Could you check a few things on this model? Use its own coordinates, in mm. Face numbers are marked on the shaded views. A direction names the side the tool comes from. Give positions to 0.01 mm unless a question says otherwise; leave off trailing zeros. One line per item, written item: value.
```python
from build123d import *

# Parameters (mm, degrees)
CUT_EXTRUDE2_OUTLINE_R = 47.625
CUT_EXTRUDE2_DEPTH     = 7.234682
F_10_CLEARANCE_HOLE1_D = 5.1054
CIRPATTERN1_COUNT      = 8
CLEARANCING_START      = -7.234682
SKETCH25_R             = 66.675
CLEARANCING_DEPTH      = 7.234682


# Read off the part's stored shape, not the designer's step: Cut-Extrude2
with BuildPart() as part:
    # Sketch24 → Revolve1 (revolve)
    with BuildSketch(Plane(origin=(0, 0, 0), x_dir=(1, 0, 0), z_dir=(0, 1, 0))):
        Polygon((-17.018, -22.86), (-17.018, -8.923782), (-34.42208, -8.923782), (-34.42208, 0), (-47.625, 0), (-47.625, -7.234682), (-46.0375, -7.234682), (-46.0375, -10.371582), (-50.8, -10.371582), (-50.8, -7.234682), (-66.675, -7.234682), (-66.675, -22.86), align=None)
    revolve(axis=Axis((0, 0, -9.275318), (0, 0, 1)))

    # Cut-Extrude2 outline → Cut-Extrude2 (cut)
    with BuildSketch(Plane.XY):
        Circle(CUT_EXTRUDE2_OUTLINE_R)
        with BuildLine():
            add(Edge.make_bspline(
                [(35.948703812, 0), (35.9515816, 0.07538119), (35.957337916, 0.226162951), (35.964207937, 0.452426553), (35.969771157, 0.678783022), (35.978029534, 1.131847853), (35.980843708, 2.190601907), (35.920311441, 3.779931016), (35.747323363, 5.668216834), (35.489928088, 7.474298946), (35.141459932, 9.268877369), (34.702390603, 11.047358984), (34.17343386, 12.80516853), (33.555538624, 14.537761538), (32.849887572, 16.240636382), (32.057893687, 17.909346365), (31.181197352, 19.53951152), (30.221662701, 21.126830276), (29.181373626, 22.667090912), (28.062629225, 24.156182809), (26.867938753, 25.590107465), (25.60001603, 26.964989265), (24.261773335, 28.277085961), (22.856314773, 29.522798851), (21.386929147, 30.698682629), (19.85708232, 31.801454876), (18.270409111, 32.828005175), (16.630704717, 33.775403815), (14.941915703, 34.640910073), (13.208130556, 35.421980041), (11.43356985, 36.116273987), (9.622576022, 36.721663214), (7.779602801, 37.236236415), (5.909204301, 37.658305492), (4.016023818, 37.986410831), (2.104782347, 38.219326014), (0.180266852, 38.356061949), (-1.75268168, 38.395870413), (-3.689180377, 38.338246992), (-5.624316777, 38.182933409), (-7.553161251, 37.929919231), (-9.470779522, 37.579442948), (-11.37224525, 37.131992419), (-13.252652651, 36.588304682), (-15.107129112, 35.949365124), (-16.930847778, 35.216406011), (-18.719040078, 34.390904381), (-20.467008144, 33.474579298), (-22.170137115, 32.469388481), (-23.823907266, 31.377524301), (-25.42390596, 30.201409162), (-26.965839357, 28.943690275), (-28.445543888, 27.607233836), (-29.858997424, 26.195118613), (-31.202330147, 24.710628968), (-32.471835063, 23.157247319), (-33.663978152, 21.538646066), (-34.775408104, 19.858679), (-35.802965645, 18.121372202), (-36.743692396, 16.330914471), (-37.594839261, 14.491647299), (-38.353874308, 12.608054401), (-39.018490139, 10.68475085), (-39.586610697, 8.726471825), (-40.056397525, 6.738061006), (-40.426255434, 4.724458642), (-40.694837576, 2.690689328), (-40.861049894, 0.641849508), (-40.924054953, -1.416905249), (-40.883275123, -3.480373184), (-40.738395114, -5.543319447), (-40.489363842, -7.600489337), (-40.13639564, -9.646621653), (-39.679970776, -11.676462103), (-39.120835312, -13.684776759), (-38.460000265, -15.666365517), (-37.698740094, -17.61607551), (-36.838590511, -19.528814477), (-35.881345602, -21.399564006), (-34.829054288, -23.223392663), (-33.684016107, -24.995468936), (-32.44877635, -26.711073982), (-31.126120537, -28.365614138), (-29.719068263, -29.954633155), (-28.230866416, -31.473824138), (-26.664981791, -32.919041144), (-25.025093105, -34.286310417), (-23.315082441, -35.571841228), (-21.53902614, -36.772036288), (-19.701185153, -37.883501708), (-17.805994889, -38.903056478), (-15.85805457, -39.827741435), (-13.862116128, -40.654827709), (-11.823072667, -41.381824596), (-9.745946518, -42.006486871), (-7.635876912, -42.526821485), (-5.498107312, -42.941093656), (-3.337972426, -43.247832311), (-1.160884928, -43.445834888), (1.027678058, -43.534171454), (3.222188708, -43.512188152), (5.417082419, -43.379509955), (7.606771886, -43.136042707), (9.785661288, -42.781974466), (11.948160555, -42.317776118), (14.08869967, -41.74420128), (16.201742982, -41.062285471), (18.281803484, -40.273344558), (20.323457017, -39.378972487), (22.321356376, -38.381038284), (24.27024527, -37.281682345), (26.164972102, -36.083312015), (28.000503535, -34.788596469), (29.77193781, -33.400460899), (31.474517775, -31.92208003), (33.103643596, -30.356870964), (34.654885111, -28.708485383), (36.123993806, -26.980801118), (37.506914359, -25.17791311), (38.799795742, -23.304123775), (39.999001844, -21.363932809), (41.101121576, -19.362026441), (41.938186302, -17.641904891), (42.402189205, -16.588613759), (42.554027377, -16.231646763)],
                knots=[0, 0, 0, 0, 0.000879209, 0.001758645, 0.002638305, 0.003518191, 0.007039982, 0.014977213, 0.022047939, 0.029133237, 0.036233164, 0.043347773, 0.050477114, 0.057621232, 0.06478017, 0.071953969, 0.079142669, 0.086346306, 0.093564916, 0.100798534, 0.108047194, 0.115310927, 0.122589766, 0.12988374, 0.13719288, 0.144517215, 0.151856774, 0.159211583, 0.16658167, 0.173967063, 0.181367786, 0.188783866, 0.196215328, 0.203662198, 0.211124498, 0.218602253, 0.226095488, 0.233604225, 0.241128486, 0.248668296, 0.256223676, 0.263794648, 0.271381234, 0.278983456, 0.286601335, 0.294234891, 0.301884146, 0.309549121, 0.317229835, 0.324926308, 0.332638561, 0.340366614, 0.348110485, 0.355870195, 0.363645762, 0.371437205, 0.379244543, 0.387067795, 0.39490698, 0.402762115, 0.410633219, 0.41852031, 0.426423405, 0.434342523, 0.442277682, 0.450228898, 0.458196189, 0.466179572, 0.474179065, 0.482194684, 0.490226447, 0.498274369, 0.506338468, 0.514418761, 0.522515263, 0.530627991, 0.538756962, 0.546902191, 0.555063694, 0.563241488, 0.571435588, 0.57964601, 0.58787277, 0.596115883, 0.604375364, 0.61265123, 0.620943495, 0.629252175, 0.637577285, 0.64591884, 0.654276855, 0.662651345, 0.671042324, 0.679449808, 0.687873812, 0.696314349, 0.704771435, 0.713245083, 0.721735309, 0.730242127, 0.738765551, 0.747305595, 0.755862273, 0.7644356, 0.77302559, 0.781632256, 0.790255613, 0.798895674, 0.807552454, 0.816225965, 0.824916222, 0.833623239, 0.842347028, 0.851087604, 0.859844979, 0.868619169, 0.877410184, 0.88621804, 0.895042749, 0.903884325, 0.912742781, 0.921618129, 0.930510383, 0.935031581, 0.935031581, 0.935031581, 0.935031581], degree=3))
            ThreePointArc((35.948703812, 0), (36.836858206, -3.871377871), (39.552581276, -6.769865934))
            ThreePointArc((39.552581276, -6.769865934), (42.805320101, -10.94498561), (42.554027377, -16.231646763))
        make_face(mode=Mode.SUBTRACT)
    extrude(amount=CUT_EXTRUDE2_DEPTH, mode=Mode.SUBTRACT)

    # #10 Clearance Hole1 (through all)
    with Locations(Plane(origin=(55.733032799, -23.085378057, 7.234682), x_dir=(-1, 0, 0), z_dir=(0, 0, -1))):
        with Locations((0, 0)):
            f_10_clearance_hole1 = Hole(F_10_CLEARANCE_HOLE1_D / 2)

    # CirPattern1: #10 Clearance Hole1 ×8 about axis
    cirpattern1_axis = Axis((0, 0, 0), (0, 0, 1))
    for i in range(1, CIRPATTERN1_COUNT):
        add(f_10_clearance_hole1.rotate(cirpattern1_axis, i * 360 / CIRPATTERN1_COUNT), mode=Mode.SUBTRACT)

    # Sketch25 → Clearancing (cut)
    with BuildSketch(Plane(origin=(0, 0, 0), x_dir=(-1, 0, 0), z_dir=(0, 0, -1)).offset(CLEARANCING_START)):
        Circle(SKETCH25_R)
        with BuildLine():
            ThreePointArc((-39.485738347, -6.87785215), (-42.684264858, -10.983386498), (-42.437160346, -16.181936632))
            add(Edge.make_bspline(
                [(-42.437160346, -16.181936632), (-41.450328446, -18.501948894), (-40.287188075, -20.70386066), (-37.62426385, -24.882183045), (-36.1244575, -26.858578596), (-33.612918368, -29.647784963), (-32.727511557, -30.551787217), (-30.899288351, -32.26713978), (-29.954285679, -33.081629815), (-27.028415852, -35.398073541), (-24.957331886, -36.773902575), (-22.214143518, -38.277928099), (-21.657736444, -38.567871448), (-20.529077868, -39.125607363), (-19.957869924, -39.392805227), (-18.236811973, -40.153613466), (-17.074606136, -40.608998857), (-13.544408375, -41.82291337), (-11.1331575, -42.430323242), (-8.045152005, -42.931279628), (-7.423828634, -43.018467653), (-6.17358737, -43.166313281), (-5.545687994, -43.226778512), (-3.668882092, -43.366672694), (-2.421130233, -43.405411027), (1.311985825, -43.361475459), (3.787286298, -43.119848136), (7.47956464, -42.43089353), (8.712476258, -42.144649273), (11.128372813, -41.470614218), (12.31452175, -41.08278751), (15.808874803, -39.769919796), (18.053477953, -38.696639775), (21.289209419, -36.780985477), (22.349089848, -36.088250708), (24.383348169, -34.625595136), (25.362502881, -33.853290457), (28.188051648, -31.415612474), (29.923427118, -29.630442917), (31.900539288, -27.191684875), (32.287236817, -26.69215724), (33.03483793, -25.679954076), (33.395921295, -25.167211132), (34.441621812, -23.609372602), (35.088773016, -22.544710991), (36.882357275, -19.273503621), (37.882174946, -16.990390194), (38.875744828, -14.00270068), (39.061155114, -13.399331831), (39.402369545, -12.191519857), (39.558676578, -11.585611614), (39.985275792, -9.761961138), (40.441402975, -7.314651304), (40.674139412, -4.836063161), (40.763559938, -2.965202227), (40.779154388, -2.339591952), (40.781417609, -1.08432134), (40.76799572, -0.453052442), (40.627903307, 2.692390804), (40.286121576, 5.161443437), (39.43890774, 8.796132878), (39.100388573, 9.996140785), (38.308399323, 12.37248564), (37.852097598, 13.554391573), (36.333140039, 16.997228128), (35.119491675, 19.170506242), (33.001368487, 22.2498484), (32.245396403, 23.246004252), (31.033998954, 24.693258097), (30.616682544, 25.168342498), (29.765008734, 26.092546286), (29.329638676, 26.542937105), (27.105848432, 28.737227444), (25.177853658, 30.309665479), (22.580283298, 32.044782733), (22.051311937, 32.380188303), (20.974087609, 33.027312806), (20.424315753, 33.339806048), (18.760945416, 34.232685111), (17.631513907, 34.770110987), (14.183245166, 36.213360105), (11.805002439, 36.951757683), (8.729750366, 37.586018139), (8.107774126, 37.698555851), (6.863218919, 37.892276195), (6.240962177, 37.973521872), (4.374253461, 38.171221637), (1.88547224, 38.31227114), (-0.602985761, 38.211399864), (-2.469206159, 38.043607473), (-3.091259068, 37.972290691), (-4.335323004, 37.798308656), (-4.959105867, 37.695274824), (-8.05217871, 37.104825218), (-10.442064996, 36.396124759), (-13.903223174, 34.987468388), (-15.036178129, 34.459888971), (-16.703458261, 33.578668593), (-17.255286668, 33.26900823), (-18.337021034, 32.625547889), (-18.867738625, 32.291418051), (-21.471435266, 30.559817088), (-23.396215015, 28.98129219), (-25.602702171, 26.764423917), (-26.03392942, 26.30874761), (-26.875809699, 25.372259656), (-27.286623762, 24.891064324), (-28.473720562, 23.426447254), (-29.209796712, 22.416679591), (-31.255817918, 19.289573594), (-32.405286999, 17.075476116), (-33.791719154, 13.550670272), (-34.189829991, 12.359597052), (-34.85899573, 9.95467515), (-35.402182987, 7.524154989), (-35.69403317, 5.042564271), (-35.815892674, 3.161655555), (-35.840306869, 2.530241223), (-35.855853683, 1.267408077), (-35.845894895, 0.636088005), (-35.821796258, 0.004844883)],
                knots=[0, 0, 0, 0, 0.03125, 0.03125, 0.0625, 0.0625, 0.078125, 0.078125, 0.09375, 0.09375, 0.125, 0.125, 0.1328125, 0.1328125, 0.140625, 0.140625, 0.15625, 0.15625, 0.1875, 0.1875, 0.1953125, 0.1953125, 0.203125, 0.203125, 0.21875, 0.21875, 0.25, 0.25, 0.265625, 0.265625, 0.28125, 0.28125, 0.3125, 0.3125, 0.328125, 0.328125, 0.34375, 0.34375, 0.375, 0.375, 0.3828125, 0.3828125, 0.390625, 0.390625, 0.40625, 0.40625, 0.4375, 0.4375, 0.4453125, 0.4453125, 0.453125, 0.453125, 0.46875, 0.484375, 0.484375, 0.4921875, 0.4921875, 0.5, 0.5, 0.53125, 0.53125, 0.546875, 0.546875, 0.5625, 0.5625, 0.59375, 0.59375, 0.609375, 0.609375, 0.6171875, 0.6171875, 0.625, 0.625, 0.65625, 0.65625, 0.6640625, 0.6640625, 0.671875, 0.671875, 0.6875, 0.6875, 0.71875, 0.71875, 0.7265625, 0.7265625, 0.734375, 0.734375, 0.75, 0.765625, 0.765625, 0.7734375, 0.7734375, 0.78125, 0.78125, 0.8125, 0.8125, 0.828125, 0.828125, 0.8359375, 0.8359375, 0.84375, 0.84375, 0.875, 0.875, 0.8828125, 0.8828125, 0.890625, 0.890625, 0.90625, 0.90625, 0.9375, 0.9375, 0.953125, 0.953125, 0.96875, 0.984375, 0.984375, 0.9921875, 0.9921875, 1, 1, 1, 1], degree=3))
            ThreePointArc((-35.821796258, 0.004844883), (-36.724753226, -3.931055952), (-39.485738347, -6.87785215))
        make_face(mode=Mode.SUBTRACT)
    extrude(amount=CLEARANCING_DEPTH, mode=Mode.SUBTRACT)


solid = part.part
```
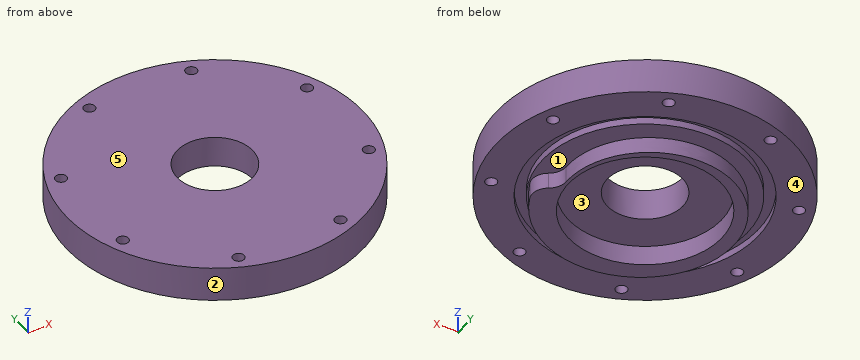
1) Suppose I cut it at A-A, the plane z = 17.5. State how many separate pieces and enclosed holes the cut face has, then the cut area to 3 significant figures.
Answer below:
separate pieces: 1
enclosed holes: 9
area: 12,900 mm2
2) We'd pull the mould along X, two halves only. Please class the marked faces 1, 2 and 3: +X half, -X half, draft (parallel to the pull), parting line (faces both ways), or undercut.
Answer below:
face 1: draft
face 2: parting line
face 3: undercut
3) For the marked faces 4 and 5, which set-ups out of +Z, -Z, +X, -X, +Y, -Y let a thin tool reach every point of the face, with its end or its side?
Answer below:
face 4: -Z
face 5: +Z, +X, -X, +Y, -Y
4) For P1, Ø6, axis at x = 32.5, z = 5.5, coming from the -Y side; P2, Ø3, axis at y = 17.5, z = 19.5, coming from the +X side; P3, Ø12, axis at y = -33, z = 19.5, coming from the +X side, each with a flat end and sliding along its axis, tell me the tip position at first contact or that it passes through.
Answer below:
P1: stops at y = -59.52
P2: stops at x = 64.73
P3: stops at x = 60.96
5) If I drill on line 1 along X through (y, z) = (-54, 19); line 2 along X through (y, z) = (-27.5, 9); line 3 along X through (y, z) = (0, 4), over which ranges is the centre line in solid material (lowest first)?
Answer below:
line 1: x = -39.11 to -24.96, -21.21 to 21.21, 24.96 to 39.11
line 2: x = -60.74 to -42.71, -36.92 to 36.92, 42.71 to 60.74
line 3: x = -40.75 to -34.42, 34.42 to 35.82
